from build123d import *

# Parameters (mm, degrees)
F0_W     = 120
F0_H     = 120
F0_R     = 1.6
F1_DEPTH = 6
F2_W     = 120
F2_H     = 120
F3_DEPTH = 0.6


with BuildPart() as f1:
    # F0 (on Top) → F1 (new body)
    with BuildSketch(Plane.XY):
        Rectangle(F0_W, F0_H)
        with Locations((-52.72189, -51.956826)):
            Circle(F0_R, mode=Mode.SUBTRACT)
        with Locations((-37.72189, -51.956826)):
            Circle(F0_R, mode=Mode.SUBTRACT)
        with Locations((-52.72189, -36.956826)):
            Circle(F0_R, mode=Mode.SUBTRACT)
        with Locations((-37.72189, -36.956826)):
            Circle(F0_R, mode=Mode.SUBTRACT)
        with Locations((-22.72189, -51.956826)):
            Circle(F0_R, mode=Mode.SUBTRACT)
        with Locations((-7.72189, -51.956826)):
            Circle(F0_R, mode=Mode.SUBTRACT)
        with Locations((-22.72189, -36.956826)):
            Circle(F0_R, mode=Mode.SUBTRACT)
        with Locations((-7.72189, -36.956826)):
            Circle(F0_R, mode=Mode.SUBTRACT)
        with Locations((-52.72189, -21.956826)):
            Circle(F0_R, mode=Mode.SUBTRACT)
        with Locations((-37.72189, -21.956826)):
            Circle(F0_R, mode=Mode.SUBTRACT)
        with Locations((-52.72189, -6.956826)):
            Circle(F0_R, mode=Mode.SUBTRACT)
        with Locations((-37.72189, -6.956826)):
            Circle(F0_R, mode=Mode.SUBTRACT)
        with Locations((-22.72189, -21.956826)):
            Circle(F0_R, mode=Mode.SUBTRACT)
        with Locations((-7.72189, -21.956826)):
            Circle(F0_R, mode=Mode.SUBTRACT)
        with Locations((-22.72189, -6.956826)):
            Circle(F0_R, mode=Mode.SUBTRACT)
        with Locations((-7.72189, -6.956826)):
            Circle(F0_R, mode=Mode.SUBTRACT)
        with Locations((7.27811, -51.956826)):
            Circle(F0_R, mode=Mode.SUBTRACT)
        with Locations((22.27811, -51.956826)):
            Circle(F0_R, mode=Mode.SUBTRACT)
        with Locations((7.27811, -36.956826)):
            Circle(F0_R, mode=Mode.SUBTRACT)
        with Locations((22.27811, -36.956826)):
            Circle(F0_R, mode=Mode.SUBTRACT)
        with Locations((37.27811, -51.956826)):
            Circle(F0_R, mode=Mode.SUBTRACT)
        with Locations((52.27811, -51.956826)):
            Circle(F0_R, mode=Mode.SUBTRACT)
        with Locations((37.27811, -36.956826)):
            Circle(F0_R, mode=Mode.SUBTRACT)
        with Locations((52.27811, -36.956826)):
            Circle(F0_R, mode=Mode.SUBTRACT)
        with Locations((7.27811, -21.956826)):
            Circle(F0_R, mode=Mode.SUBTRACT)
        with Locations((22.27811, -21.956826)):
            Circle(F0_R, mode=Mode.SUBTRACT)
        with Locations((7.27811, -6.956826)):
            Circle(F0_R, mode=Mode.SUBTRACT)
        with Locations((22.27811, -6.956826)):
            Circle(F0_R, mode=Mode.SUBTRACT)
        with Locations((37.27811, -21.956826)):
            Circle(F0_R, mode=Mode.SUBTRACT)
        with Locations((52.27811, -21.956826)):
            Circle(F0_R, mode=Mode.SUBTRACT)
        with Locations((37.27811, -6.956826)):
            Circle(F0_R, mode=Mode.SUBTRACT)
        with Locations((52.27811, -6.956826)):
            Circle(F0_R, mode=Mode.SUBTRACT)
        with Locations((-52.72189, 8.043174)):
            Circle(F0_R, mode=Mode.SUBTRACT)
        with Locations((-37.72189, 8.043174)):
            Circle(F0_R, mode=Mode.SUBTRACT)
        with Locations((-52.72189, 23.043174)):
            Circle(F0_R, mode=Mode.SUBTRACT)
        with Locations((-37.72189, 23.043174)):
            Circle(F0_R, mode=Mode.SUBTRACT)
        with Locations((-22.72189, 8.043174)):
            Circle(F0_R, mode=Mode.SUBTRACT)
        with Locations((-7.72189, 8.043174)):
            Circle(F0_R, mode=Mode.SUBTRACT)
        with Locations((-22.72189, 23.043174)):
            Circle(F0_R, mode=Mode.SUBTRACT)
        with Locations((-7.72189, 23.043174)):
            Circle(F0_R, mode=Mode.SUBTRACT)
        with Locations((-52.72189, 38.043174)):
            Circle(F0_R, mode=Mode.SUBTRACT)
        with Locations((-37.72189, 38.043174)):
            Circle(F0_R, mode=Mode.SUBTRACT)
        with Locations((-52.72189, 53.043174)):
            Circle(F0_R, mode=Mode.SUBTRACT)
        with Locations((-37.72189, 53.043174)):
            Circle(F0_R, mode=Mode.SUBTRACT)
        with Locations((-22.72189, 38.043174)):
            Circle(F0_R, mode=Mode.SUBTRACT)
        with Locations((-7.72189, 38.043174)):
            Circle(F0_R, mode=Mode.SUBTRACT)
        with Locations((-22.72189, 53.043174)):
            Circle(F0_R, mode=Mode.SUBTRACT)
        with Locations((-7.72189, 53.043174)):
            Circle(F0_R, mode=Mode.SUBTRACT)
        with Locations((7.27811, 8.043174)):
            Circle(F0_R, mode=Mode.SUBTRACT)
        with Locations((22.27811, 8.043174)):
            Circle(F0_R, mode=Mode.SUBTRACT)
        with Locations((7.27811, 23.043174)):
            Circle(F0_R, mode=Mode.SUBTRACT)
        with Locations((22.27811, 23.043174)):
            Circle(F0_R, mode=Mode.SUBTRACT)
        with Locations((37.27811, 8.043174)):
            Circle(F0_R, mode=Mode.SUBTRACT)
        with Locations((52.27811, 8.043174)):
            Circle(F0_R, mode=Mode.SUBTRACT)
        with Locations((37.27811, 23.043174)):
            Circle(F0_R, mode=Mode.SUBTRACT)
        with Locations((52.27811, 23.043174)):
            Circle(F0_R, mode=Mode.SUBTRACT)
        with Locations((7.27811, 38.043174)):
            Circle(F0_R, mode=Mode.SUBTRACT)
        with Locations((22.27811, 38.043174)):
            Circle(F0_R, mode=Mode.SUBTRACT)
        with Locations((7.27811, 53.043174)):
            Circle(F0_R, mode=Mode.SUBTRACT)
        with Locations((22.27811, 53.043174)):
            Circle(F0_R, mode=Mode.SUBTRACT)
        with Locations((37.27811, 38.043174)):
            Circle(F0_R, mode=Mode.SUBTRACT)
        with Locations((52.27811, 38.043174)):
            Circle(F0_R, mode=Mode.SUBTRACT)
        with Locations((37.27811, 53.043174)):
            Circle(F0_R, mode=Mode.SUBTRACT)
        with Locations((52.27811, 53.043174)):
            Circle(F0_R, mode=Mode.SUBTRACT)
    extrude(amount=F1_DEPTH)

    # F2 (on face) → F3 (join)
    with BuildSketch(Plane(origin=(0, 0, 0), x_dir=(1, 0, 0), z_dir=(0, 0, -1))):
        Rectangle(F2_W, F2_H)
    extrude(amount=F3_DEPTH)


solid = f1.part
Model file for the job. Use its own axes, mm. Round coordinates to 2 decimals unless told otherwise and drop trailing zeros. Write each question's results on one line, items separated by ' | '. Start each with the question number.
(1) Probe probe 1 along Z at (x, y) = (38.5, -52.5). List the from-to ranges inside material, lowest first. Write a range as from..to.
(2) Drop flat-ended pins along their axis: pin 1 (3.5 mm diameter, centred on x = 7.28, y = 23.04, fed in from +Z); pin 2 (1 mm diameter, centred on x = -52.5, y = -37.5, fed in from +Z). Give the stop position or say it passes through.
(3) Saw through at A-A, the plane z = 5. State how many separate pieces and enclosed holes the cut face has, then the cut area to 3 significant figures.
Established:
1) probe 1: z = -0.6..0
2) pin 1: stops at z = 6 | pin 2: stops at z = 0
3) separate pieces: 1 | enclosed holes: 64 | area: 13,900 mm^2
